Part model, mm, in its own coordinate system. Face numbers are marked on the shaded views. A direction names the side the tool comes from. Round coordinates to 2 decimals unless told otherwise and drop trailing zeros. Order: outer loops, then holes, each group sorted by start corner. A loop starts at its lowest first (then second) coordinate and runs counter-clockwise, first axis right, second up. Notation, with made-up numbers: (-7.75, 26) - (12.25, 26) arc R11 ccw to (12.25, 35) - close; hole circle Ø5 at (58.25, -34.75). An arc over 180 degrees is marked (long way). Return JSON: item names as keys, results as strings. Group by question number.
Item 1: Saw through at B-B on z = 4.05. List the corners of the cut face in (x, y), and give its area (3 significant figures).
Item 2: Probe probe 1 along X at (y, z) = (13.3, 2.9); probe 2 along X at (y, z) = (6.16, 1.55); probe 3 along Y at (x, z) = (63, 2.95). List the from-to ranges inside material, lowest first.
Item 3: Drop flat-ended pins along their axis: pin 1 (3 mm diameter, centred on x = 63.04, y = 13.2, fed in from +Z); pin 2 (2.5 mm diameter, centred on y = 22, z = 3.5, fed in from -X); pin 3 (1.6 mm diameter, centred on x = 4.5, z = 3, fed in from +Y); pin 4 (3 mm diameter, centred on y = 22.5, z = 1, fed in from +X). Give the stop position or say it passes through.
Item 4: Two-plate mould, pull along Y, no slides. Class the marked faces 1, 2 and 3: released by +Y, released by -Y, zero draft, split by the parting line, or undercut.
Item 5: Tool access for the marked faces 4, 5 and 6: list every direction of +Z, -Z, +X, -X, +Y, -Y with a clear straight run to the whole face (end or side of a thin tool).
Item 6: Saw through at A-A on y = 23.75. List the corners of the cut face in (x, z).
Item 7: Saw through at C-C on x = 35. List the corners of the cut face in (y, z).
```python
from build123d import *

# Parameters (mm, degrees)
MODEL_R             = 4.75
MODEL_R_2           = 3.95
MODEL_R_3           = 1.2
BOSS_EXTRUDE1_DEPTH = 5.35


with BuildPart() as part:
    # Model → Boss-Extrude1 (new body)
    with BuildSketch(Plane.XY):
        Polygon((0, 19.999999553), (0, 0), (70.000000298, 0), (70.000000298, 19.999999553), (56.000001729, 19.999999553), (56.000001729, 25.349999778), (41.999999434, 25.349999778), (41.999999434, 19.999999553), (28.000000864, 19.999999553), (28.000000864, 25.349999778), (14.000000432, 25.349999778), (14.000000432, 19.999999553), align=None)
        with Locations((35, 5.999999553)):
            Circle(MODEL_R, mode=Mode.SUBTRACT)
        with Locations((63, 5.999999553)):
            Circle(MODEL_R_2, mode=Mode.SUBTRACT)
        with Locations((7, 5.999999553)):
            Circle(MODEL_R_2, mode=Mode.SUBTRACT)
        with Locations((14, 6.159999553)):
            Circle(MODEL_R_3, mode=Mode.SUBTRACT)
        with Locations((56, 6.159999553)):
            Circle(MODEL_R_3, mode=Mode.SUBTRACT)
        with Locations((63.04, 13.199999553)):
            Circle(MODEL_R_3, mode=Mode.SUBTRACT)
        with Locations((7.29808245, 13.299999553)):
            Circle(MODEL_R_3, mode=Mode.SUBTRACT)
    extrude(amount=BOSS_EXTRUDE1_DEPTH)


solid = part.part
```
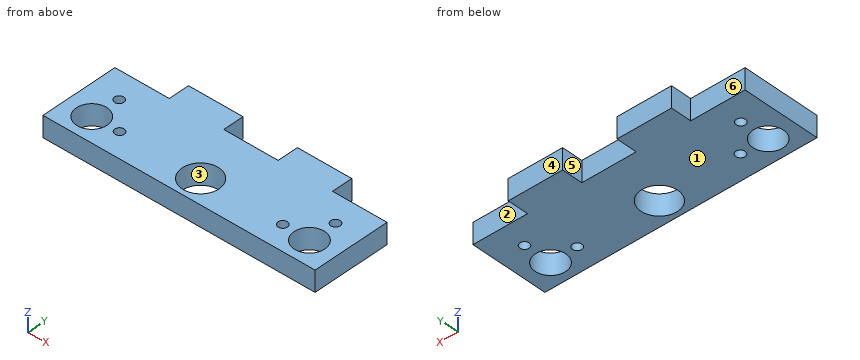
Filled in:
{
 "1": {"outline": "(0, 0) - (70, 0) - (70, 20) - (56, 20) - (56, 25.35) - (42, 25.35) - (42, 20) - (28, 20) - (28, 25.35) - (14, 25.35) - (14, 20) - (0, 20) - close; hole circle Ø7.9 at (7, 6); hole circle Ø2.4 at (7.3, 13.3); hole circle Ø2.4 at (14, 6.16); hole circle Ø9.5 at (35, 6); hole circle Ø2.4 at (56, 6.16); hole circle Ø7.9 at (63, 6); hole circle Ø2.4 at (63.04, 13.2)", "area": "1,360 mm^2"},
 "2": {"probe 1": "x = 0 to 6.1, 8.5 to 61.84, 64.24 to 70", "probe 2": "x = 0 to 3.05, 10.95 to 12.8, 15.2 to 30.25, 39.75 to 54.8, 57.2 to 59.05, 66.95 to 70", "probe 3": "y = 0 to 2.05, 9.95 to 12, 14.4 to 20"},
 "3": {"pin 1": "stops at z = 5.35", "pin 2": "stops at x = 14", "pin 3": "stops at y = 20", "pin 4": "stops at x = 56"},
 "4": {"face 1": "zero draft", "face 2": "released by +Y", "face 3": "undercut"},
 "5": {"face 4": "+Z, -Z, +X, -X, +Y", "face 5": "+Z, -Z, +Y", "face 6": "+Z, -Z, -X, +Y"},
 "6": {"outline": "(14, 0) - (28, 0) - (28, 5.35) - (14, 5.35) - close; (42, 0) - (56, 0) - (56, 5.35) - (42, 5.35) - close"},
 "7": {"outline": "(0, 0) - (1.25, 0) - (1.25, 5.35) - (0, 5.35) - close; (10.75, 0) - (20, 0) - (20, 5.35) - (10.75, 5.35) - close"}
}
